```python
from build123d import *

# Parameters (mm, degrees)
F0_R     = 20
F0_R_2   = 6
F1_DEPTH = 25


with BuildPart() as f1:
    # F0 (on Front) → F1 (new body)
    with BuildSketch(Plane.XZ):
        with BuildLine():
            Line((-50, -31), (0, -31))
            ThreePointArc((0, -31), (5.026517, -30.589772), (9.92, -29.369944))
            Line((9.92, -29.369944), (54.8, -14.211263))
            ThreePointArc((54.8, -14.211263), (65, 0), (54.8, 14.211263))
            Line((54.8, 14.211263), (9.92, 29.369944))
            ThreePointArc((9.92, 29.369944), (-8.790322, 29.727601), (-24.297307, 19.252036))
            ThreePointArc((-24.297307, 19.252036), (-30.975734, 17.312857), (-35.000008, 22.984455))
            ThreePointArc((-35.000008, 22.984455), (-49.992227, 37.999998), (-65, 23))
            Line((-65, 23), (-65, -16))
            ThreePointArc((-65, -16), (-60.606602, -26.606602), (-50, -31))
        make_face()
        Circle(F0_R, mode=Mode.SUBTRACT)
        with Locations((50, 0)):
            Circle(F0_R_2, mode=Mode.SUBTRACT)
        with BuildLine():
            ThreePointArc((-57, 23), (-50, 30), (-43, 23))
            Line((-43, 23), (-43, -16))
            ThreePointArc((-43, -16), (-50, -23), (-57, -16))
            Line((-57, -16), (-57, 23))
        make_face(mode=Mode.SUBTRACT)
    extrude(amount=F1_DEPTH)


solid = f1.part
```
For this review, take the finished solid that the model builds, in its own axes (mm). A direction names the side the tool comes from. Give positions to 0.01 mm unless a question says otherwise; leave off trailing zeros. Write each loop counter-clockwise with the first axis right and the second up, starting at its lowest first coordinate (ties: lowest second). Pieces come first, ordered by that corner, then holes. Notation, with made-up numbers: M 8.5,13.25 L 64.5,13.25 A17 ccw 64.5,24.25 Z; hole C -26.5,67.5 d7. An arc over 180 degrees is marked long. One line per item, written item: value.
1) The part is to be moulded in two halves that separate along X. For faces 1 (the flat face through (32.674, -12.325, 21.684)), 2 (the flat face through (-15, 0, -19)), 3 (the cylindrical face through (-50, -12, 30)), 4 (the flat face through (-65, -12, 4)), say which applies: +X half, -X half, draft (parallel to the pull), parting line (faces both ways), or undercut.
Results are:
face 1: +X half
face 2: draft
face 3: undercut
face 4: -X half
2) Take a section at B-B, the plane y = -4.5. Write out the cut boundary in (x, z).
Results are:
outline: M -65,-16 A15 ccw -50,-31 L 0,-31 A31 ccw 9.92,-29.37 L 54.8,-14.21 A15 ccw 54.8,14.21 L 9.92,29.37 A31 ccw -24.3,19.25 A6 cw -35,22.98 A15 ccw -65,23 Z; hole M -57,-16 A7 ccw -43,-16 L -43,23 A7 ccw -57,23 Z; hole C 0,0 d40; hole C 50,0 d12
3) For line 1 (Z direction, x = 0, y = -6); line 2 (X direction, y = -8, z = -7.5); line 3 (X direction, y = -7.5, z = 10), list the stretches that pass through material, from the lowest coordinate up. Write a range as from..to.
Results are:
line 1: z = -31..-20, 20..31
line 2: x = -65..-57, -43..-18.54, 18.54..62.99
line 3: x = -65..-57, -43..-17.32, 17.32..61.18
4) Take a section at C-C, the plane x = 50. Write out the cut boundary in (y, z), then the cut area to 3 significant figures.
Results are:
outline: M -25,-15.83 L 0,-15.83 L 0,-6 L -25,-6 Z; M -25,6 L 0,6 L 0,15.83 L -25,15.83 Z
area: 492 mm²
5) For P1, Ø8, axis at x = 27, y = -19.5, coming from the +Z side; P2, Ø3, axis at y = -6.5, z = -6.5, coming from the +X side; P3, Ø15.5, axis at x = 50, z = 0, coming from the +Y side; P4, Ø1, axis at x = 15.5, y = -13, coming from the -Z side, all flat-tipped, find the tip position at first contact; note any pin that passes through.
Results are:
P1: stops at z = 24.95
P2: stops at x = 64.14
P3: stops at y = 0
P4: stops at z = -27.65
6) For faces 5 (the flat face through (-43, -12, 4)), 6 (the cylindrical face through (65, -12, 0)), list the 3-axis set-ups (+Z, -Z, +X, -X, +Y, -Y) from which the entire face can be reached by the end or side of a thin tool; tool diameter is ignored.
Results are:
face 5: +Y, -Y
face 6: +X, +Y, -Y
7) Take a section at D-D, the plane z = 0. Write out the cut boundary in (x, y).
Results are:
outline: M -65,-25 L -57,-25 L -57,0 L -65,0 Z; M -43,-25 L -20,-25 L -20,0 L -43,0 Z; M 20,-25 L 44,-25 L 44,0 L 20,0 Z; M 56,-25 L 65,-25 L 65,0 L 56,0 Z
8) Take a section at A-A, the plane z = 12. Write out the cut boundary in (x, y).
Results are:
outline: M -65,-25 L -57,-25 L -57,0 L -65,0 Z; M -43,-25 L -16,-25 L -16,0 L -43,0 Z; M 16,-25 L 59,-25 L 59,0 L 16,0 Z
